Read the model definition and answer for the solid it produces. Units are mm, in the model's axes. Face numbers are marked on the shaded views. A direction names the side the tool comes from. Coordinates: 2 decimals unless noted, no trailing zeros. Write each loop counter-clockwise with the first axis right and the second up, starting at its lowest first coordinate (ties: lowest second). Pieces come first, ordered by that corner, then holes. Notation, with made-up numbers: (-3, 26.25) -> (51, 26.25) arc R18 cw to (51, 45.25) -> close; hole circle Ø1 at (56, 56). An arc over 180 degrees is marked (long way). Use CSV: the item, a comma, the result in double quotes. Start each with the question number.
from build123d import *

# Parameters (mm, degrees)
F0_W      = 80
F0_H      = 8
F1_DEPTH  = 21
F3_DEPTH  = 25
F5_DEPTH  = 2.5
F7_DEPTH  = 2.5
F8_R      = 5
F9_W      = 80
F9_H      = 20
F10_DEPTH = 9
F11_R     = 2
F12_DEPTH = 25
F13_R     = 3
F14_DEPTH = 5
F15_R     = 2.5
F16_DEPTH = 25


with BuildPart() as f1:
    # F0 (on Top) → F1 (new body)
    with BuildSketch(Plane.XY):
        with Locations((40, 4)):
            Rectangle(F0_W, F0_H)
    extrude(amount=F1_DEPTH)

    # F2 (on face) → F3 (cut)
    with BuildSketch(Plane.XZ):
        with BuildLine():
            Line((37.5, 21), (37.5, 15))
            ThreePointArc((37.5, 15), (40, 12.5), (42.5, 15))
            Line((42.5, 15), (42.5, 21))
            Line((42.5, 21), (37.5, 21))
        make_face()
    extrude(amount=-F3_DEPTH, mode=Mode.SUBTRACT)

    # F4 (on face) → F5 (cut)
    with BuildSketch(Plane.XZ):
        with BuildLine():
            Line((36, 21), (36, 15))
            ThreePointArc((36, 15), (40, 11), (44, 15))
            Line((44, 15), (44, 21))
            Line((44, 21), (42.5, 21))
            Line((42.5, 21), (42.5, 15))
            ThreePointArc((42.5, 15), (40, 12.5), (37.5, 15))
            Line((37.5, 15), (37.5, 21))
            Line((37.5, 21), (36, 21))
        make_face()
    extrude(amount=-F5_DEPTH, mode=Mode.SUBTRACT)

    # F6 (on face) → F7 (cut)
    with BuildSketch(Plane(origin=(0, 8, 0), x_dir=(-1, 0, 0), z_dir=(0, 1, 0))):
        with BuildLine():
            Line((-44, 21), (-44, 15))
            ThreePointArc((-44, 15), (-40, 11), (-36, 15))
            Line((-36, 15), (-36, 21))
            Line((-36, 21), (-37.5, 21))
            Line((-37.5, 21), (-37.5, 15))
            ThreePointArc((-37.5, 15), (-40, 12.5), (-42.5, 15))
            Line((-42.5, 15), (-42.5, 21))
            Line((-42.5, 21), (-44, 21))
        make_face()
    extrude(amount=-F7_DEPTH, mode=Mode.SUBTRACT)

    # F8
    f8_edges = [f1.edges().sort_by_distance(p)[0] for p in [
        (42.5, 4, 21),
        (37.5, 4, 21),
    ]]
    fillet(f8_edges, radius=F8_R)

    # F9 (on face) → F10 (join)
    with BuildSketch(Plane(origin=(0, 0, 0), x_dir=(1, 0, 0), z_dir=(0, 0, -1))):
        with Locations((40, 2)):
            Rectangle(F9_W, F9_H)
    extrude(amount=F10_DEPTH)

    # F11 (on face) → F12 (cut)
    with BuildSketch(Plane.XY):
        with Locations((10, -6)):
            Circle(F11_R)
        with Locations((25, -6)):
            Circle(F11_R)
        with Locations((70, -6)):
            Circle(F11_R)
        with Locations((55, -6)):
            Circle(F11_R)
    extrude(amount=-F12_DEPTH, mode=Mode.SUBTRACT)

    # F13 (on face) → F14 (cut)
    with BuildSketch(Plane.XY):
        with Locations((10, -6)):
            Circle(F13_R)
        with Locations((25, -6)):
            Circle(F13_R)
        with Locations((55, -6)):
            Circle(F13_R)
        with Locations((70, -6)):
            Circle(F13_R)
    extrude(amount=-F14_DEPTH, mode=Mode.SUBTRACT)

    # F15 (on face) → F16 (cut)
    with BuildSketch(Plane.XZ):
        with Locations((12, 13.5)):
            Circle(F15_R)
    extrude(amount=-F16_DEPTH, mode=Mode.SUBTRACT)


solid = f1.part
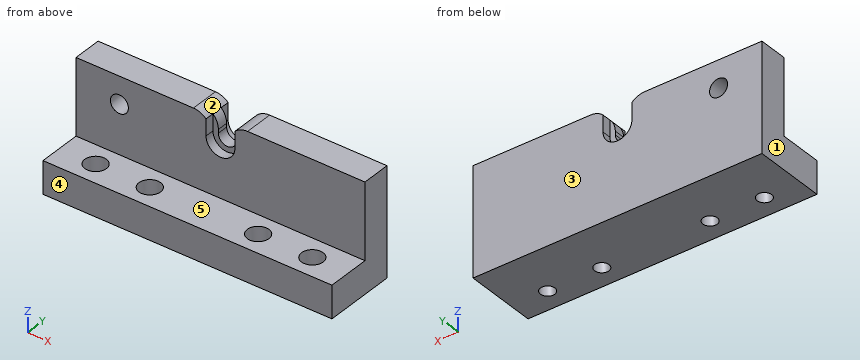
1) Find the intervals of material crossed by line 1 along X through (y, z) = (0.25, 12.25); line 2 along Y through (x, z) = (25, -2.6); line 3 along Z through (x, y) = (15.5, -1.5), in increasing order.
2) The mould has two halves that part along X. Classify the marked faces 1, 2 and 3: pulls with the +X half, pulls with the -X half, needs draft (parallel to the pull), parting line crosses it, or undercut.
3) Each of these flat-tipped pins is pushed along its axis until it touches: pin 1 (5 mm diameter, centred on x = 70, y = -5, fed in from +Z); pin 2 (5 mm diameter, centred on x = 10, y = -6, fed in from +Z); pin 3 (10.5 mm diameter, centred on x = 47, z = 7.5, fed in from -Y); pin 4 (3 mm diameter, centred on x = 12, z = 13.5, fed in from +Y). Where does it stop, or does it pass through?
4) Section C-C, the plane x = 40 is taken. Give the vertices of the cut face in (y, z).
5) Section D-D, the plane z = 13.5 is taken. Give the vertices of the cut face in (x, y).
6) Section A-A, the plane y = 3.75 is taken. Give the vertices of the cut face in (x, z), plus the area to 3 significant figures.
7) Which of the six approach directions +Z, -Z, +X, -X, +Y, -Y give full straight-line access (tool end or side, diameter ignored) to the marked faces 4 and 5?
8) Section B-B, the plane x = 70 is taken. Give the vertices of the cut face in (y, z).
The answers:
1,line 1,"x = 0 to 9.83, 14.17 to 37.1, 42.9 to 80"
1,line 2,"y = -12 to -9, -3 to 8"
1,line 3,"z = -9 to 0"
2,face 1,"pulls with the -X half"
2,face 2,"undercut"
2,face 3,"needs draft"
3,pin 1,"stops at z = 0"
3,pin 2,"stops at z = -5"
3,pin 3,"stops at y = 0"
3,pin 4,"passes through"
4,outline,"(-12, -9) -> (8, -9) -> (8, 11) -> (5.5, 11) -> (5.5, 12.5) -> (2.5, 12.5) -> (2.5, 11) -> (0, 11) -> (0, 0) -> (-12, 0) -> close"
5,outline,"(0, 0) -> (9.5, 0) -> (9.5, 8) -> (0, 8) -> close; (14.5, 0) -> (36.29, 0) -> (36.29, 2.5) -> (38, 2.5) -> (38, 5.5) -> (36.29, 5.5) -> (36.29, 8) -> (14.5, 8) -> close; (42, 2.5) -> (43.71, 2.5) -> (43.71, 0) -> (80, 0) -> (80, 8) -> (43.71, 8) -> (43.71, 5.5) -> (42, 5.5) -> close"
6,outline,"(0, -9) -> (80, -9) -> (80, 21) -> (47.5, 21) arc R5 ccw to (42.5, 16) -> (42.5, 15) arc R2.5 cw to (37.5, 15) -> (37.5, 16) arc R5 ccw to (32.5, 21) -> (0, 21) -> close; hole circle Ø5 at (12, 13.5)"
6,area,"2,330 mm^2"
7,face 4,"+Z, -Z, +X, -X, -Y"
7,face 5,"+Z, +X, -X, -Y"
8,outline,"(-12, -9) -> (-8, -9) -> (-8, -5) -> (-9, -5) -> (-9, 0) -> (-12, 0) -> close; (-4, -9) -> (8, -9) -> (8, 21) -> (0, 21) -> (0, 0) -> (-3, 0) -> (-3, -5) -> (-4, -5) -> close"
